Verification items for the finished model (mm, model axes). Give positions to 0.01 mm unless a question says otherwise; leave off trailing zeros. Order: outer loops, then holes, each group sorted by start corner. A loop starts at its lowest first (then second) coordinate and runs counter-clockwise, first axis right, second up. Notation, with made-up numbers: (68.5, 68.5) -> (88.5, 68.5) arc R24 cw to (88.5, 107.5) -> close; hole circle Ø6 at (87, 34). An arc over 180 degrees is marked (long way). Return JSON: item names as keys, results as strings. Group by question number.
(1) Thickness scan on line 1 along Z through (x, y) = (-1, 0.75); line 2 along Z through (x, y) = (6, 3.25); line 3 along X through (y, z) = (4.75, -1.5). Record the ranges inside material, lowest first.
(2) Release check for a two-part mould opening along X. For faces 1 (the face through (-3.998, 0.61, 12.696)), 2 (the face through (-10, 0, -1)), 3 (the face through (5.371, 2.09, -7.005)) record: pulls with the +X half, pulls with the -X half, needs draft (parallel to the pull), parting line crosses it, or undercut.
(3) Cross-section at B-B on x = 0. Enter the section's corners in (y, z) (3 decimals), then the cut area to 3 significant figures.
(4) Cross-section at C-C on y = 5. Enter the section's corners in (x, z), then the cut area to 3 significant figures.
(5) Cross-section at D-D on y = 3.25. Enter the section's corners in (x, z).
(6) Depth check by flat-ended pin: pin 1 Ø3 at (y, z) = (5.5, 12) entering from -X; pin 2 Ø5 at (x, z) = (-2, 4) entering from -Y (3 decimals); pin 3 Ø3 at (x, y) = (7, 1.5) entering from +Z; pin 4 Ø3 at (x, y) = (7.5, 4) entering from +Z. Enter the tip coordinate at first touch or a pass-through.
(7) Cross-section at A-A on z = 0. Enter the section's corners in (x, y) (3 decimals).
from build123d import *

# Parameters (mm, degrees)
FILLET1_R = 1.27


with BuildPart() as part:
    # Sketch1 → Revolve1 (revolve)
    with BuildSketch(Plane.XY, mode=Mode.PRIVATE) as revolve1_sk:
        Polygon((-12.7, 0), (-19.05, 6.35), (-11.286174209, 6.35), (-7.62, 0), align=None)
    revolve(revolve1_sk.sketch.rotate(Axis((0, 6.6675, 0), (0, -1, 0)), 270), axis=Axis((0, 6.6675, 0), (0, -1, 0)))

    # Fillet1
    fillet1_edges = [part.edges().sort_by_distance(p)[0] for p in [
        (0, 0, -12.7),
        (0, 6.35, -19.05),
        (0, 6.35, -11.286174209),
        (0, 0, -7.62),
    ]]
    fillet(fillet1_edges, radius=FILLET1_R)


solid = part.part
Verdict:
{
 "1": {"line 1": "-13.41 to -8.6, 8.6 to 13.41", "line 2": "-14.78 to -7.36, 7.36 to 14.78", "line 3": "-17.14 to -10.25, 10.25 to 17.14"},
 "2": {"face 1": "parting line crosses it", "face 2": "needs draft", "face 3": "undercut"},
 "3": {"outline": "(0, -12.174) arc R1.27 ccw to (0.372, -13.072) -> (4.182, -16.882) arc R1.27 ccw to (6.35, -15.984) -> (6.35, -12.019) arc R1.27 ccw to (5.715, -10.92) -> (1.905, -8.72) arc R1.27 ccw to (0, -9.82) -> close; (0, 9.82) arc R1.27 ccw to (1.905, 8.72) -> (5.715, 10.92) arc R1.27 ccw to (6.35, 12.019) -> (6.35, 15.984) arc R1.27 ccw to (4.182, 16.882) -> (0.372, 13.072) arc R1.27 ccw to (0, 12.174) -> close", "area": "75.1 mm²"},
 "4": {"outline": "circle Ø34.5 at (0, 0); hole circle Ø21.01 at (0, 0)", "area": "588 mm²"},
 "5": {"outline": "circle Ø31.9 at (0, 0); hole circle Ø18.99 at (0, 0)"},
 "6": {"pin 1": "x = -13.66", "pin 2": "through", "pin 3": "z = 14.2", "pin 4": "z = 16.06"},
 "7": {"outline": "(-16.882, 4.182) -> (-13.072, 0.372) arc R1.27 ccw to (-12.174, 0) -> (-9.82, 0) arc R1.27 ccw to (-8.72, 1.905) -> (-10.92, 5.715) arc R1.27 ccw to (-12.019, 6.35) -> (-15.984, 6.35) arc R1.27 ccw to start; (8.72, 1.905) arc R1.27 ccw to (9.82, 0) -> (12.174, 0) arc R1.27 ccw to (13.072, 0.372) -> (16.882, 4.182) arc R1.27 ccw to (15.984, 6.35) -> (12.019, 6.35) arc R1.27 ccw to (10.92, 5.715) -> close"}
}
